Read the model definition and answer for the solid it produces. Units are mm, in the model's axes. A direction names the side the tool comes from. Give positions to 0.01 mm unless a question says otherwise; leave off trailing zeros. Write each loop counter-clockwise with the first axis right and the second up, starting at its lowest first coordinate (ties: lowest second). Pieces come first, ordered by that corner, then holes. Notation, with made-up numbers: M -32.75,48 L 0.25,48 A15 ccw 0.25,59 Z; hole C 19,76.25 d1. An arc over 180 degrees is marked long. Put each result on its own line as item: value.
from build123d import *

# Parameters (mm, degrees)
SKETCH_R     = 4.2
PAD006_DEPTH = 1.5
SKETCH012_R  = 3
PAD007_DEPTH = 3
POCKET_DEPTH = 0.2


with BuildPart() as part:
    # Sketch → Pad006 (new body)
    with BuildSketch(Plane.XY.offset(29.2)):
        with Locations((14.8, -53.5)):
            Circle(SKETCH_R)
    extrude(amount=-PAD006_DEPTH)

    # Sketch012 (on Face2 of Pad006) → Pad007 (join)
    with BuildSketch(Plane.XY.offset(29.2)):
        with Locations((14.8, -53.5)):
            Circle(SKETCH012_R)
    extrude(amount=PAD007_DEPTH)

    # Sketch013 (on Face5 of Pad007) → Pocket (cut)
    with BuildSketch(Plane.XY.offset(32.2)):
        with BuildLine():
            ThreePointArc((15.86066, -52.43934), (13.3, -53.5), (15.86066, -54.56066))
            ThreePointArc((16.426344, -55.126347), (16.426345, -54.560662), (15.86066, -54.56066))
            ThreePointArc((16.426348, -51.873657), (12.5, -53.499997), (16.426344, -55.126347))
            ThreePointArc((15.86066, -52.43934), (16.426346, -52.439343), (16.426348, -51.873657))
        make_face()
        with BuildLine():
            ThreePointArc((14.8, -53.1), (14.4, -53.5), (14.8, -53.9))
            Line((14.8, -53.9), (17, -53.9))
            ThreePointArc((17, -53.9), (17.4, -53.5), (17, -53.1))
            Line((14.8, -53.1), (17, -53.1))
        make_face()
    extrude(amount=-POCKET_DEPTH, mode=Mode.SUBTRACT)


solid = part.part
(1) Section C-C on z = 31.75 is taken. Determine the outline of the cut face in (x, y), and give its area (3 significant figures).
Result:
outline: C 14.8,-53.5 d6
area: 28.3 mm²
(2) For a pull along Y with two mould halves and no side action, classify faces 3 (the face through (17, -56, 29.2)), 4 (the face through (13, -53, 32)), 5 (the face through (11.704, -50.661, 28.46)) as +Y half, -Y half, draft (parallel to the pull), parting line (faces both ways), or undercut.
Result:
face 3: draft
face 4: undercut
face 5: parting line
(3) Straight lines are drawn through the part: line 1 along Y through (x, z) = (14.8, 32.1); line 2 along Z through (x, y) = (13.5, -56.75); line 3 along Z through (x, y) = (13.75, -55). For each, find the intervals that lie inside material, in ascending order. Write a range as from..to.
Result:
line 1: y = -56.5..-55.8, -55..-53.9, -53.1..-52, -51.2..-50.5
line 2: z = 27.7..29.2
line 3: z = 27.7..32
(4) Section B-B on x = 16 is taken. Determine the outline of the cut face in (y, z).
Result:
outline: M -57.52,27.7 L -49.48,27.7 L -49.48,29.2 L -50.75,29.2 L -50.75,32.2 L -51.54,32.2 L -51.54,32 L -52.53,32 L -52.53,32.2 L -53.1,32.2 L -53.1,32 L -53.9,32 L -53.9,32.2 L -54.47,32.2 L -54.47,32 L -55.46,32 L -55.46,32.2 L -56.25,32.2 L -56.25,29.2 L -57.52,29.2 Z
(5) Section D-D on y = -54.75 is taken. Determine the outline of the cut face in (x, z).
Result:
outline: M 10.79,27.7 L 18.81,27.7 L 18.81,29.2 L 17.53,29.2 L 17.53,32.2 L 16.53,32.2 L 16.53,32 L 15.63,32 L 15.63,32.2 L 13.97,32.2 L 13.97,32 L 12.87,32 L 12.87,32.2 L 12.07,32.2 L 12.07,29.2 L 10.79,29.2 Z
(6) Which of the six approach directions +Z, -Z, +X, -X, +Y, -Y give full straight-line access (tool end or side, diameter ignored) to faces 1 (the face through (14.409, -50.526, 30.679)), 2 (the face through (15, -53, 27.7))?
Result:
face 1: +Z
face 2: -Z, +X, -X, +Y, -Y
(7) Section A-A on y = -53.5 is taken. Determine the outline of the cut face in (x, z).
Result:
outline: M 10.6,27.7 L 19,27.7 L 19,29.2 L 17.8,29.2 L 17.8,32.2 L 17.4,32.2 L 17.4,32 L 14.4,32 L 14.4,32.2 L 13.3,32.2 L 13.3,32 L 12.5,32 L 12.5,32.2 L 11.8,32.2 L 11.8,29.2 L 10.6,29.2 Z
(8) Given pin 1 Ø1 at (y, z) = (-50.5, 29) entering from +X; pin 2 Ø1 at (x, z) = (15, 31) entering from -Y; pin 3 Ø1 at (x, z) = (16, 28) entering from -Y, each flat-ended and moving along its own axis, determine where each tip first touches the part or whether it passes through.
Result:
pin 1: stops at x = 18.17
pin 2: stops at y = -56.5
pin 3: stops at y = -57.64
